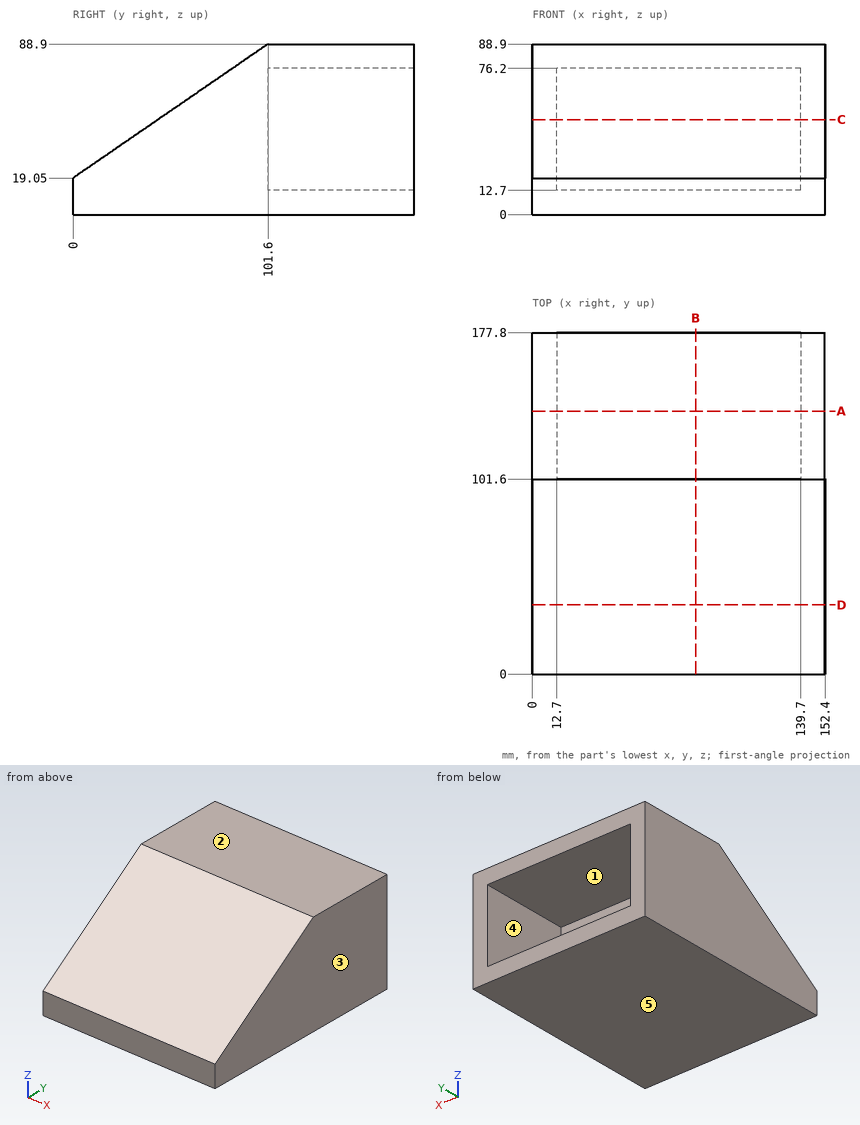
Verification items for this drawing (mm, ordinates from the low corner). A direction names the side the tool comes from. Give positions to 0.01 mm unless a question says otherwise; leave off trailing zeros. Write each loop counter-clockwise with the first axis right and the second up, starting at its lowest first coordinate (ties: lowest second). Pieces come first, ordered by that corner, then holes. Notation, with made-up numbers: (-3, -17) -> (56, -17) arc R29 ccw to (56, 22) -> close; hole circle Ø6 at (3, 10). An arc over 180 degrees is marked (long way). Use one line per item in the form item = value.
Item 1: Sectioned sample at A-A on y = 137. Enter the section's corners in (x, z).
Results list:
outline = (0, 0) -> (152.4, 0) -> (152.4, 88.9) -> (0, 88.9) -> close; hole (12.7, 12.7) -> (139.7, 12.7) -> (139.7, 76.2) -> (12.7, 76.2) -> close
Item 2: Sectioned sample at C-C on z = 49.5. Enter the section's corners in (x, y), plus the area to 3 significant figures.
Results list:
outline = (0, 44.29) -> (152.4, 44.29) -> (152.4, 177.8) -> (139.7, 177.8) -> (139.7, 101.6) -> (12.7, 101.6) -> (12.7, 177.8) -> (0, 177.8) -> close
area = 10,700 mm2
Item 3: Access from +Z, -Z, +X, -X, +Y, -Y to the whole of each face (thin tool, end or side, straight path). Record for the marked faces 1 and 2.
Results list:
face_1 = +Y
face_2 = +Z, +X, -X, +Y, -Y
Item 4: Depth check by flat-ended pin: pin 1 Ø1 at (x, z) = (50, 74) entering from +Y; pin 2 Ø1 at (x, z) = (124, 74.5) entering from -Y; pin 3 Ø4 at (x, y) = (107.5, 40) entering from +Z (3 decimals). Enter the tip coordinate at first touch or a pass-through.
Results list:
pin_1 = 101.6
pin_2 = 79.93
pin_3 = 47.925
Item 5: Sectioned sample at B-B on x = 85. Enter the section's corners in (y, z).
Results list:
outline = (0, 0) -> (177.8, 0) -> (177.8, 12.7) -> (101.6, 12.7) -> (101.6, 76.2) -> (177.8, 76.2) -> (177.8, 88.9) -> (101.6, 88.9) -> (0, 19.05) -> close
Item 6: Scan lines: line 1 (Z direction, x = 114.5, y = 127.5); line 2 (X direction, y = 159, z = 38); line 3 (Y direction, x = 81, z = 59.5). Record each from-to range of solid material in increasing order.
Results list:
line_1 = 0 to 12.7, 76.2 to 88.9
line_2 = 0 to 12.7, 139.7 to 152.4
line_3 = 58.84 to 101.6
Item 7: Sectioned sample at D-D on y = 36. Enter the section's corners in (x, z), plus the area to 3 significant figures.
Results list:
outline = (0, 0) -> (152.4, 0) -> (152.4, 43.8) -> (0, 43.8) -> close
area = 6,680 mm2
Item 8: Mould release check, pull along X, two halves, no side actions. Record for the marked faces 3, 4 and 5: released by +X, released by -X, zero draft, split by the parting line, or undercut.
Results list:
face_3 = released by +X
face_4 = undercut
face_5 = zero draft
